Read the model definition and answer for the solid it produces. Units are mm, in the model's axes. A direction names the side the tool comes from. Give positions to 0.01 mm unless a question says otherwise; leave off trailing zeros. Write each loop counter-clockwise with the first axis right and the second up, starting at its lowest first coordinate (ties: lowest second). Pieces come first, ordered by that corner, then holes.
```python
from build123d import *

# Parameters (mm, degrees)
F0_R          = 7
F1_DEPTH      = 2.8
F2_R          = 5.875
F3_DEPTH      = 5
F4_R          = 1.25
F5_DEPTH      = 7.001
F5_DEPTH_BACK = 7.001
F6_R          = 2.5
F7_DEPTH      = 6.1


with BuildPart() as f1:
    # F0 (on Top) → F1 (new body)
    with BuildSketch(Plane.XY):
        Circle(F0_R)
    extrude(amount=F1_DEPTH)

    # F2 (on face) → F3 (join)
    with BuildSketch(Plane.XY.offset(2.8)):
        Circle(F2_R)
    extrude(amount=F3_DEPTH)

    # F4 (on Front) → F5 (cut, two sides)
    with BuildSketch(Plane.XZ) as f5_sk:
        with Locations((0, 1.1)):
            Circle(F4_R)
    extrude(amount=-F5_DEPTH, mode=Mode.SUBTRACT)
    extrude(f5_sk.sketch, amount=F5_DEPTH_BACK, mode=Mode.SUBTRACT)

    # F6 (on face) → F7 (cut, through all)
    with BuildSketch(Plane.XY.offset(7.8)):
        Circle(F6_R)
    extrude(amount=-F7_DEPTH, mode=Mode.SUBTRACT)


solid = f1.part
```
Item 1: Section A-A (y = 0) is taken. Write down the section's boundary in (x, z) (3 decimals).
Result set:
outline: (-7, 0) - (-0.594, 0) arc R1.25 cw to (-1.097, 1.7) - (-2.5, 1.7) - (-2.5, 7.8) - (-5.875, 7.8) - (-5.875, 2.8) - (-7, 2.8) - close; (0.594, 0) - (7, 0) - (7, 2.8) - (5.875, 2.8) - (5.875, 7.8) - (2.5, 7.8) - (2.5, 1.7) - (1.097, 1.7) arc R1.25 cw to start
Item 2: Section B-B (x = 0) is taken. Write down the section's boundary in (y, z) (3 decimals), and give its area (3 significant figures).
Result set:
outline: (-7, 2.35) - (-2.5, 2.35) - (-2.5, 7.8) - (-5.875, 7.8) - (-5.875, 2.8) - (-7, 2.8) - close; (2.5, 2.35) - (7, 2.35) - (7, 2.8) - (5.875, 2.8) - (5.875, 7.8) - (2.5, 7.8) - close
area: 37.8 mm2
Item 3: Which of the six approach directions +Z, -Z, +X, -X, +Y, -Y give full straight-line access (tool end or side, diameter ignored) to faces 4 (the cylindrical face through (1.17, -0.1, 1.54)), 5 (the flat face through (-2, 0, 1.7))?
Result set:
face 4: +Y, -Y
face 5: +Z
Item 4: Find the intervals of material crossed by line 1 along X through (y, z) = (0.25, 1.1); line 2 along Z through (x, y) = (1.5, -6.25); line 3 along Y through (x, z) = (-1.75, 5), in increasing order.
Result set:
line 1: x = -7 to -1.25, 1.25 to 7
line 2: z = 0 to 2.8
line 3: y = -5.61 to -1.79, 1.79 to 5.61
Item 5: Each of these flat-tipped pins is pushed along its axis until it touches: pin 1 Ø1 at (y, z) = (3.5, 5.5) entering from -X; pin 2 Ø1.5 at (x, y) = (-1.5, 0) entering from +Z; pin 3 Ø1.5 at (x, z) = (3.5, 3) entering from -Y; pin 4 Ø2 at (x, z) = (0, 1.1) entering from +Y. Where does it stop, or does it pass through?
Result set:
pin 1: stops at x = -5.05
pin 2: stops at z = 1.7
pin 3: stops at y = -6.43
pin 4: passes through
Item 6: Section C-C (z = 7) is taken. Write down the section's boundary in (x, y) (3 decimals).
Result set:
outline: circle Ø11.75 at (0, 0); hole circle Ø5 at (0, 0)
Item 7: Determine the mould class of faces 1 (the flat face through (-2, 6, 2.8)), 2 (the cylindrical face through (3.23, -6.21, 1.38)), 3 (the cylindrical face through (2.385, 0.751, 4.793)) for opening direction X: pulls with the +X half, pulls with the -X half, needs draft (parallel to the pull), parting line crosses it, or undercut.
Result set:
face 1: needs draft
face 2: parting line crosses it
face 3: undercut
Item 8: Section D-D (y = -4.5) is taken. Write down the section's boundary in (x, z).
Result set:
outline: (-5.36, 0) - (-0.59, 0) arc R1.25 cw (long way) to (0.59, 0) - (5.36, 0) - (5.36, 2.8) - (3.78, 2.8) - (3.78, 7.8) - (-3.78, 7.8) - (-3.78, 2.8) - (-5.36, 2.8) - close
